For this review, take the finished solid that the model builds, in its own axes (mm). Face numbers are marked on the shaded views. A direction names the side the tool comes from. Round coordinates to 2 decimals unless told otherwise and drop trailing zeros. Order: outer loops, then holes, each group sorted by start corner. A loop starts at its lowest first (then second) coordinate and runs counter-clockwise, first axis right, second up. Notation, with made-up numbers: (72.5, 56) -> (126.5, 56) arc R14 cw to (126.5, 73) -> close; hole circle Ø4 at (37.5, -17). An arc over 180 degrees is marked (long way). Use a Markdown table: item, result. Add a question column.
1) Consider section A-A (z = 3). State the section outline as (x, y) points, plus the area to 3 significant figures.
2) Wall thickness on line 1 along Z through (x, y) = (11.75, -1.5); line 2 along Y through (x, z) = (4.25, 3.3); line 3 along X through (y, z) = (-14.25, 0.65): over which ranges is each line inside the solid? List them lowest first. Write a range as [from, to].
3) Consider section D-D (x = 13.25). State the section outline as (y, z) points.
4) Clearance check with flat-ended pins moving along their axes: P1, Ø3, axis at y = -11.5, z = 4, coming from the +X side; P2, Ø1.2, axis at x = 11.75, z = 3, coming from the -Y side; P3, Ø3, axis at x = 11, z = 4.5, coming from the -Y side. State where each tip first meets the part, or that it passes through.
5) Machinability: for the marked faces 1 and 2, which of the approach directions +Z, -Z, +X, -X, +Y, -Y give a long, thin tool a straight path to every point of the face, cutting with its end or side? Answer none if there is none.
6) Draft analysis for pull direction X (two halves, no side actions). For the marked faces 3, 4, 5 and 6, state which applies: pulls with the +X half, pulls with the -X half, needs draft (parallel to the pull), parting line crosses it, or undercut.
7) Consider section B-B (y = -13.75). State the section outline as (x, z) points, plus the area to 3 significant figures.
8) Consider section C-C (x = 11.75). State the section outline as (y, z) points.
```python
from build123d import *

# Parameters (mm, degrees)
F0_W     = 14.75
F0_H     = 6
F0_R     = 1
F1_DEPTH = 2
F2_W     = 2
F2_H     = 6
F3_DEPTH = 14.75
F4_R     = 1
F5_DEPTH = 25


with BuildPart() as f1:
    # F0 (on Front) → F1 (new body)
    with BuildSketch(Plane.XZ):
        with Locations((7.375, 3)):
            Rectangle(F0_W, F0_H)
        with Locations((11.75, 3)):
            Circle(F0_R, mode=Mode.SUBTRACT)
    extrude(amount=F1_DEPTH)

    # F2 (on face) → F3 (join)
    with BuildSketch(Plane.XZ.offset(2)):
        with Locations((1, 3)):
            Rectangle(F2_W, F2_H)
    extrude(amount=F3_DEPTH)

    # F4 (on face) → F5 (cut)
    with BuildSketch(Plane.YZ.offset(2)):
        with Locations((-13.75, 3)):
            Circle(F4_R)
    extrude(amount=-F5_DEPTH, mode=Mode.SUBTRACT)


solid = f1.part
```
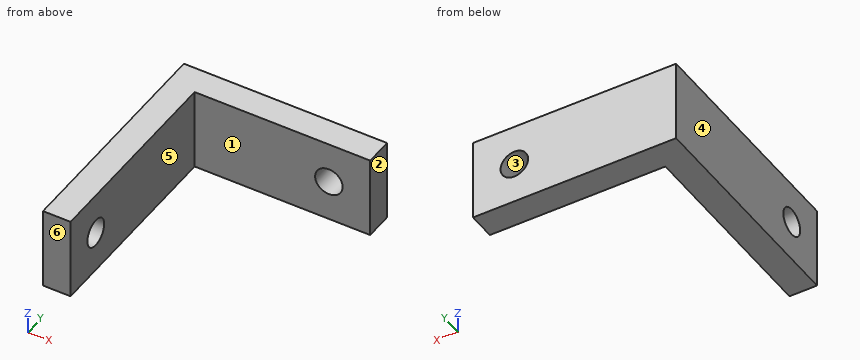
Results list:
| question | item | result |
|---|---|---|
| 1 | outline | (0, -16.75) -> (2, -16.75) -> (2, -14.75) -> (0, -14.75) -> close; (0, -12.75) -> (2, -12.75) -> (2, -2) -> (10.75, -2) -> (10.75, 0) -> (0, 0) -> close; (12.75, -2) -> (14.75, -2) -> (14.75, 0) -> (12.75, 0) -> close |
| 1 | area | 51.0 mm2 |
| 2 | line 1 | [0, 2], [4, 6] |
| 2 | line 2 | [-2, 0] |
| 2 | line 3 | [0, 2] |
| 3 | outline | (-2, 0) -> (0, 0) -> (0, 6) -> (-2, 6) -> close |
| 4 | P1 | x = 2 |
| 4 | P2 | through |
| 4 | P3 | y = -2 |
| 5 | face 1 | +Z, -Z, +X, -Y |
| 5 | face 2 | +Z, -Z, +X, +Y, -Y |
| 6 | face 3 | undercut |
| 6 | face 4 | pulls with the -X half |
| 6 | face 5 | pulls with the +X half |
| 6 | face 6 | needs draft |
| 7 | outline | (0, 0) -> (2, 0) -> (2, 2) -> (0, 2) -> close; (0, 4) -> (2, 4) -> (2, 6) -> (0, 6) -> close |
| 7 | area | 8.00 mm2 |
| 8 | outline | (-2, 0) -> (0, 0) -> (0, 2) -> (-2, 2) -> close; (-2, 4) -> (0, 4) -> (0, 6) -> (-2, 6) -> close |
